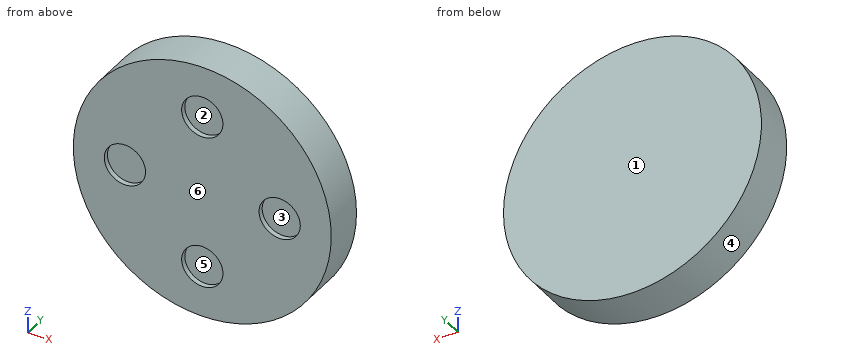
```python
from build123d import *

# Parameters (mm, degrees)
F0_R     = 250
F1_DEPTH = 80
F2_R     = 40
F3_DEPTH = 10


with BuildPart() as f1:
    # F0 (on Front) → F1 (new body)
    with BuildSketch(Plane.XZ):
        Circle(F0_R)
    extrude(amount=F1_DEPTH)

    # F2 (on face) → F3 (cut)
    with BuildSketch(Plane.XZ.offset(80)):
        with Locations((0, 150)):
            Circle(F2_R)
        with Locations((-150, 0)):
            Circle(F2_R)
        with Locations((0, -150)):
            Circle(F2_R)
        with Locations((150, 0)):
            Circle(F2_R)
    extrude(amount=-F3_DEPTH, mode=Mode.SUBTRACT)


solid = f1.part
```
The model under review builds one solid part; all positions refer to its coordinate system, in mm. Face numbers are marked on the shaded views. A direction names the side the tool comes from. Give positions to 0.01 mm unless a question says otherwise; leave off trailing zeros. Write each loop counter-clockwise with the first axis right and the second up, starting at its lowest first coordinate (ties: lowest second). Pieces come first, ordered by that corner, then holes. Notation, with made-up numbers: (83.5, 31) -> (113.5, 31) arc R13 ccw to (113.5, 45) -> close; hole circle Ø6 at (41.25, 73). An arc over 180 degrees is marked (long way). Answer in a Markdown table with one row per item.
1) Add section D-D on x = 150. State the section outline as (y, z) points.
Worked answers:
| item | result |
|---|---|
| outline | (-80, -200) -> (0, -200) -> (0, 200) -> (-80, 200) -> (-80, 40) -> (-70, 40) -> (-70, -40) -> (-80, -40) -> close |
2) Mouldability with a two-part tool opening along X and no side actions: class the marked faces 3, 4, 5 and 6 as +X half, -X half, draft (parallel to the pull), parting line (faces both ways), or undercut.
Worked answers:
| item | result |
|---|---|
| face 3 | undercut |
| face 4 | parting line |
| face 5 | undercut |
| face 6 | draft |
3) Add section B-B on z = 0. State the section outline as (x, y) points.
Worked answers:
| item | result |
|---|---|
| outline | (-250, -80) -> (-190, -80) -> (-190, -70) -> (-110, -70) -> (-110, -80) -> (110, -80) -> (110, -70) -> (190, -70) -> (190, -80) -> (250, -80) -> (250, 0) -> (-250, 0) -> close |
4) For L1, parallel to Z at x = 0, y = -72.75; L2, parallel to Y at x = 5, z = 185; L3, parallel to Z at x = 150, y = -76, list the stretches that pass through material, from the lowest coordinate up. Write a range as [from, to].
Worked answers:
| item | result |
|---|---|
| L1 | [-250, -190], [-110, 110], [190, 250] |
| L2 | [-70, 0] |
| L3 | [-200, -40], [40, 200] |
5) Tool access review of the marked faces 1 and 2: name each direction out of +Z, -Z, +X, -X, +Y, -Y from which nothing blocks a thin tool from reaching the whole face with its end or side.
Worked answers:
| item | result |
|---|---|
| face 1 | +Z, -Z, +X, -X, +Y |
| face 2 | -Y |
6) Add section A-A on x = 0. State the section outline as (y, z) points, plus the area to 3 significant figures.
Worked answers:
| item | result |
|---|---|
| outline | (-80, -250) -> (0, -250) -> (0, 250) -> (-80, 250) -> (-80, 190) -> (-70, 190) -> (-70, 110) -> (-80, 110) -> (-80, -110) -> (-70, -110) -> (-70, -190) -> (-80, -190) -> close |
| area | 38,400 mm² |
7) Clearance check with flat-ended pins moving along their axes: P1, Ø1, axis at y = -49, z = 140, coming from the -X side; P2, Ø24, axis at x = 169.5, z = -19.5, coming from the -Y side; P3, Ø3, axis at x = 29, y = -13.5, coming from the +Z side. State where each tip first meets the part, or that it passes through.
Worked answers:
| item | result |
|---|---|
| P1 | x = -207.46 |
| P2 | y = -70 |
| P3 | z = 248.48 |
8) Add section C-C on y = -36. State the section outline as (x, z) points.
Worked answers:
| item | result |
|---|---|
| outline | circle Ø500 at (0, 0) |
